from build123d import *

# Parameters (mm, degrees)
SKETCH1_W           = 93
SKETCH1_H           = 57
BOSS_EXTRUDE1_DEPTH = 14
SHELL1_T            = -2
SKETCH2_W           = 91
SKETCH2_H           = 55
SKETCH2_W_2         = 89
SKETCH2_H_2         = 53
BOSS_EXTRUDE2_DEPTH = 1
FILLET2_R           = 2


with BuildPart() as part:
    # Sketch1 → Boss-Extrude1 (new body)
    with BuildSketch(Plane(origin=(0, 0, 0), x_dir=(1, 0, 0), z_dir=(0, 1, 0))):
        Rectangle(SKETCH1_W, SKETCH1_H)
    extrude(amount=BOSS_EXTRUDE1_DEPTH)

    # Shell1
    shell1_openings = [part.faces().sort_by_distance(p)[0] for p in [
        (0, 14, 0),
    ]]
    offset(amount=SHELL1_T, openings=shell1_openings, kind=Kind.INTERSECTION)

    # Sketch2 → Boss-Extrude2 (add)
    with BuildSketch(Plane(origin=(0, 14, 0), x_dir=(1, 0, 0), z_dir=(0, 1, 0))):
        Rectangle(SKETCH2_W, SKETCH2_H)
        Rectangle(SKETCH2_W_2, SKETCH2_H_2, mode=Mode.SUBTRACT)
    extrude(amount=BOSS_EXTRUDE2_DEPTH)

    # Fillet2
    fillet2_edges = [part.edges().sort_by_distance(p)[0] for p in [
        (0, 0, 28.5),
        (-46.5, 0, 0),
        (0, 0, -28.5),
        (46.5, 0, 0),
        (46.5, 7, 28.5),
        (-46.5, 7, 28.5),
        (-46.5, 7, -28.5),
        (46.5, 7, -28.5),
    ]]
    fillet(fillet2_edges, radius=FILLET2_R)


solid = part.part
The model under review builds one solid part; all positions refer to its coordinate system, in mm. A direction names the side the tool comes from. Round coordinates to 2 decimals unless told otherwise and drop trailing zeros. Write each loop counter-clockwise with the first axis right and the second up, starting at its lowest first coordinate (ties: lowest second). Pieces come first, ordered by that corner, then holes. Notation, with made-up numbers: M -33.5,23 L 21.5,23 A12 ccw 21.5,42 Z; hole C 6.5,-40 d5. An arc over 180 degrees is marked long. Use a Markdown table: item, result. Add a question column.
Q1. Insertion check: pin 1 (10 mm diameter, centred on x = -32.5, z = -0.5, fed in from +Y); pin 2 (0.5 mm diameter, centred on x = -10, y = 14.5, fed in from +Z). Each pin has a flat end and moves straight along its axis. Give the tip position at first contact, or say it passes through.
Q2. To check wall thickness, follow line 1 (Z direction, x = 9, y = 5.75); line 2 (X direction, y = 13, z = 17); line 3 (Y direction, x = 10.5, z = 5). State the ranges of each line that lie inside material, in increasing order.
Q3. Machinability: for faces 1 (the face through (-1, 0, 0)), 2 (the face through (-1, 8, 26.5)), which of the approach directions +Z, -Z, +X, -X, +Y, -Y give a long, thin tool a straight path to every point of the face, cutting with its end or side? Answer none if there is none.
Q4. The part is to be moulded in two halves that separate along X. For faces 3 (the face through (45.93, 8.08, 27.9)), 4 (the face through (-45.9, 8.08, 27.93)), 5 (the face through (44.5, 8, 0)), say which applies: pulls with the +X half, pulls with the -X half, needs draft (parallel to the pull), parting line crosses it, or undercut.
Q5. We need section C-C, the plane x = 2. State the section outline as (y, z) points.
Q6. We need section B-B, the plane z = 9. State the section outline as (x, y) points.
Q7. We need section A-A, the plane y = 3.5. State the section outline as (x, z) points.
Findings below:
| question | item | result |
|---|---|---|
| 1 | pin 1 | stops at y = 2 |
| 1 | pin 2 | stops at z = 27.5 |
| 2 | line 1 | z = -28.5 to -26.5, 26.5 to 28.5 |
| 2 | line 2 | x = -46.5 to -44.5, 44.5 to 46.5 |
| 2 | line 3 | y = 0 to 2 |
| 3 | face 1 | +Z, -Z, +X, -X, -Y |
| 3 | face 2 | +Y |
| 4 | face 3 | pulls with the +X half |
| 4 | face 4 | pulls with the -X half |
| 4 | face 5 | undercut |
| 5 | outline | M 0,-26.5 A2 ccw 2,-28.5 L 14,-28.5 L 14,-27.5 L 15,-27.5 L 15,-26.5 L 2,-26.5 L 2,26.5 L 15,26.5 L 15,27.5 L 14,27.5 L 14,28.5 L 2,28.5 A2 ccw 0,26.5 Z |
| 6 | outline | M -46.5,2 A2 ccw -44.5,0 L 44.5,0 A2 ccw 46.5,2 L 46.5,14 L 45.5,14 L 45.5,15 L 44.5,15 L 44.5,2 L -44.5,2 L -44.5,15 L -45.5,15 L -45.5,14 L -46.5,14 Z |
| 7 | outline | M -46.5,-26.5 A2 ccw -44.5,-28.5 L 44.5,-28.5 A2 ccw 46.5,-26.5 L 46.5,26.5 A2 ccw 44.5,28.5 L -44.5,28.5 A2 ccw -46.5,26.5 Z; hole M -44.5,-26.5 L 44.5,-26.5 L 44.5,26.5 L -44.5,26.5 Z |
